Build history of the part. All positions in model axes, mm. A direction names the side the tool comes from. Round coordinates to 2 decimals unless told otherwise and drop trailing zeros. Write each loop counter-clockwise with the first axis right and the second up, starting at its lowest first coordinate (ties: lowest second). Pieces come first, ordered by that corner, then holes. Notation, with made-up numbers: (63.25, 6) -> (69.25, 6) arc R35 cw to (69.25, 44) -> close; hole circle Ø2 at (24, -34). An arc over 180 degrees is marked (long way). Answer as CSV lines item,"result".
from build123d import *

# Parameters (mm, degrees)
SKETCH_1_W          = 10
SKETCH_1_H          = 10
SKETCH_1_W_2        = 8
SKETCH_1_H_2        = 8
EXTRUDE_1_DEPTH     = 25
SKETCH_3_R          = 1.6
CUT_EXTRUDE_1_DEPTH = 11
SKETCH_4_R          = 1.6
CUT_EXTRUDE_2_DEPTH = 11


with BuildPart() as part:
    # ｽｹｯﾁ1 → ﾎﾞｽ - 押し出し1 (new body, symmetric)
    with BuildSketch(Plane.XY):
        Rectangle(SKETCH_1_W, SKETCH_1_H)
        Rectangle(SKETCH_1_W_2, SKETCH_1_H_2, mode=Mode.SUBTRACT)
    extrude(amount=EXTRUDE_1_DEPTH, both=True)

    # ｽｹｯﾁ3 → ｶｯﾄ - 押し出し1 (cut, through all)
    with BuildSketch(Plane(origin=(5, 0, 0), x_dir=(0, 0, -1), z_dir=(1, 0, 0))):
        with Locations((-20, 0)):
            Circle(SKETCH_3_R)
        with Locations((20, 0)):
            Circle(SKETCH_3_R)
    extrude(amount=-CUT_EXTRUDE_1_DEPTH, mode=Mode.SUBTRACT)

    # ｽｹｯﾁ4 → ｶｯﾄ - 押し出し2 (cut, through all)
    with BuildSketch(Plane(origin=(0, 5, 0), x_dir=(1, 0, 0), z_dir=(0, 1, 0))):
        with Locations((0, -15)):
            Circle(SKETCH_4_R)
        with Locations((0, 15)):
            Circle(SKETCH_4_R)
    extrude(amount=-CUT_EXTRUDE_2_DEPTH, mode=Mode.SUBTRACT)


solid = part.part
1. Cut at D-D, the plane y = 2.5. Write the cut outline in (x, z), then the cut area to 3 significant figures.
Results found:
outline,"(-5, -25) -> (-4, -25) -> (-4, 25) -> (-5, 25) -> close; (4, -25) -> (5, -25) -> (5, 25) -> (4, 25) -> close"
area,"100 mm2"
2. Cut at A-A, the plane y = 0. Write the cut outline in (x, z).
Results found:
outline,"(-5, -25) -> (-4, -25) -> (-4, -21.6) -> (-5, -21.6) -> close; (-5, -18.4) -> (-4, -18.4) -> (-4, 18.4) -> (-5, 18.4) -> close; (-5, 21.6) -> (-4, 21.6) -> (-4, 25) -> (-5, 25) -> close; (4, -25) -> (5, -25) -> (5, -21.6) -> (4, -21.6) -> close; (4, -18.4) -> (5, -18.4) -> (5, 18.4) -> (4, 18.4) -> close; (4, 21.6) -> (5, 21.6) -> (5, 25) -> (4, 25) -> close"
3. Mould opens along Y. For faces 3 (the flat face through (0, 4, 0)), 4 (the flat face through (0, 5, 0)), 5 (the cylindrical face through (-0.208, 4.507, -16.586)) say: +Y half, -Y half, draft (parallel to the pull), parting line (faces both ways), or undercut.
Results found:
face 3,"undercut"
face 4,"+Y half"
face 5,"draft"
4. Cut at B-B, the plane z = 15. Write the cut outline in (x, y).
Results found:
outline,"(-5, -5) -> (-1.6, -5) -> (-1.6, -4) -> (-4, -4) -> (-4, 4) -> (-1.6, 4) -> (-1.6, 5) -> (-5, 5) -> close; (1.6, -5) -> (5, -5) -> (5, 5) -> (1.6, 5) -> (1.6, 4) -> (4, 4) -> (4, -4) -> (1.6, -4) -> close"
5. Cut at C-C, the plane x = 0. Write the cut outline in (y, z), then the cut area to 3 significant figures.
Results found:
outline,"(-5, -25) -> (-4, -25) -> (-4, -16.6) -> (-5, -16.6) -> close; (-5, -13.4) -> (-4, -13.4) -> (-4, 13.4) -> (-5, 13.4) -> close; (-5, 16.6) -> (-4, 16.6) -> (-4, 25) -> (-5, 25) -> close; (4, -25) -> (5, -25) -> (5, -16.6) -> (4, -16.6) -> close; (4, -13.4) -> (5, -13.4) -> (5, 13.4) -> (4, 13.4) -> close; (4, 16.6) -> (5, 16.6) -> (5, 25) -> (4, 25) -> close"
area,"87.2 mm2"
6. Probe line 1 along Z through (x, y) = (0, -4.75); line 2 along X through (y, z) = (-3, -10.5); line 3 along Y through (x, z) = (-4.35, 20). List the from-to ranges inside material, lowest first.
Results found:
line 1,"z = -25 to -16.6, -13.4 to 13.4, 16.6 to 25"
line 2,"x = -5 to -4, 4 to 5"
line 3,"y = -5 to -1.6, 1.6 to 5"
7. Which spindle directions (+Z, -Z, +X, -X, +Y, -Y) get a long thin tool onto all of the face, cutting with end or side? Do faces 1 (the flat face through (-4.5, 0.1, -25)), 2 (the flat face through (4, 0, 0)). Say none if no direction does.
Results found:
face 1,"-Z, +X, -X, +Y, -Y"
face 2,"+Z, -Z"
